Model file for the job. Use its own axes, mm. A direction names the side the tool comes from. Give positions to 0.01 mm unless a question says otherwise; leave off trailing zeros. Write each loop counter-clockwise with the first axis right and the second up, starting at its lowest first coordinate (ties: lowest second). Pieces come first, ordered by that corner, then holes. Notation, with made-up numbers: (67.25, 71.25) - (97.25, 71.25) arc R18 cw to (97.25, 91.25) - close; hole circle Ø1 at (1, 45.25). An arc over 180 degrees is marked (long way). One line per item, written item: value. Start each with the question number.
(1) Cut at A-A, the plane z = 11.25. List the corners of the cut face in (x, y).
(2) Cut at C-C, the plane y = -9.5. List the corners of the cut face in (x, z).
(3) Drop flat-ended pins along their axis: P1, Ø1.9, axis at x = -24.5, y = -4.5, coming from the +Z side; P2, Ø3.5, axis at y = -8.5, z = 6.5, coming from the +X side; P3, Ø2, axis at y = 6, z = 4, coming from the +X side. Give the stop position or say it passes through.
(4) Cut at B-B, the plane x = -8. List the corners of the cut face in (y, z).
(5) Mould opens along X. For faces 5 (the face through (22.4, -14.4, 6.3)), 6 (the face through (22.5, -2, 11)), 7 (the face through (-20.75, 3, 2)) say: pulls with the +X half, pulls with the -X half, needs draft (parallel to the pull), parting line crosses it, or undercut.
(6) Probe L1, parallel to X at y = -22.5, z = 5; L2, parallel to Y at x = -23, z = 5.1; L3, parallel to Y at x = -19, z = 9. List the from-to ranges inside material, lowest first.
(7) 3-axis set-ups, long thin cutter, end or side, ignore diameter. For faces 1 (the face through (-14, -22, 6)), 2 (the face through (-23, 3, 1)), 3 (the face through (-0.4, 20, 26.2)), 4 (the face through (20.28, 4.97, 2.54)): which of +Z, -Z, +X, -X, +Y, -Y reach the whole face in a straight line?
(8) Cut at D-D, the plane x = -23. List the corners of the cut face in (y, z).
from build123d import *

# Parameters (mm, degrees)
SKETCH_1_W             = 56
SKETCH_1_H             = 50
EXTRUDE_487_DEPTH      = 12.5
SKETCH_3_W             = 36
SKETCH_3_H             = 46
CUT_EXTRUDE_730_DEPTH  = 40.563240514
SKETCH_11_R            = 1.25
CUT_EXTRUDE_984_DEPTH  = 10
CUT_EXTRUDE_1451_DEPTH = 8
CUT_EXTRUDE_1793_REACH = 64.588
SKETCH_4_R             = 4.2
SKETCH_6_R             = 4
CUT_EXTRUDE_1930_DEPTH = 10
SKETCH_7_W             = 6.25
SKETCH_7_H             = 20.5
CUT_EXTRUDE_2129_DEPTH = 10
SKETCH_8_R             = 5.25
CUT_EXTRUDE_2306_DEPTH = 2.25
SKETCH_9_R             = 1.1
CUT_EXTRUDE_2664_DEPTH = 5.25
CUT_EXTRUDE_3061_DEPTH = 40.563240514
CHAMFER_1_SIZE         = 1
FILLET_1_R             = 1
SKETCH_12_W            = 20
SKETCH_12_H            = 1.5
CUT_EXTRUDE_3473_DEPTH = 40.563240514
FILLET_2_R             = 0.5
CUT_EXTRUDE_4198_REACH = 41.563
SKETCH_13_W            = 36
SKETCH_13_H            = 1
EXTRUDE_4558_DEPTH     = 5
FILLET_3_R             = 10
FILLET_4_R             = 1.5


with BuildPart() as part:
    # Эскиз1 → Extrude 487 (new body)
    with BuildSketch(Plane.XY):
        Rectangle(SKETCH_1_W, SKETCH_1_H)
    extrude(amount=EXTRUDE_487_DEPTH)

    # Эскиз3 → Cut-Extrude 730 (cut, through all)
    with BuildSketch(Plane.XY.offset(12.5)):
        with Locations((0, 1)):
            Rectangle(SKETCH_3_W, SKETCH_3_H)
    extrude(amount=-CUT_EXTRUDE_730_DEPTH, mode=Mode.SUBTRACT)

    # Эскиз11 → Cut-Extrude 984 (cut)
    with BuildSketch(Plane.XZ.offset(25)):
        with Locations(Location((-25, 5, 0), (0, 0, 270))):
            Circle(SKETCH_11_R)
        with Locations(Location((25, 5, 0), (0, 0, 270))):
            Circle(SKETCH_11_R)
    cut_extrude_984 = extrude(amount=-CUT_EXTRUDE_984_DEPTH, mode=Mode.SUBTRACT)

    # Mirror 1028: Cut-Extrude 984 across plane
    add(cut_extrude_984.mirror(Plane.ZX), mode=Mode.SUBTRACT)

    # Эскиз5 → Cut-Extrude 1451 (cut)
    with BuildSketch(Plane(origin=(28, 0, 0), x_dir=(0, 0, -1), z_dir=(1, 0, 0))):
        with BuildLine():
            Line((-9.688027281, 0.587538929), (-8.743079599, -12.085887362))
            ThreePointArc((-8.743079599, -12.085887362), (-6.25, -14.4), (-3.756920401, -12.085887362))
            Line((-3.756920401, -12.085887362), (-2.811972719, 0.587538929))
            ThreePointArc((-2.811972719, 0.587538929), (-6.25, 7.2), (-9.688027281, 0.587538929))
        make_face()
    extrude(amount=-CUT_EXTRUDE_1451_DEPTH, mode=Mode.SUBTRACT)

    # Эскиз4 → Cut-Extrude 1793 (cut, up to next)
    with BuildSketch(Plane(origin=(28, 0, 0), x_dir=(0, 0, -1), z_dir=(1, 0, 0)), mode=Mode.PRIVATE) as cut_extrude_1793_sk1:
        with Locations((-6.25, 3)):
            Circle(SKETCH_4_R)
    cut_extrude_1793_tool1 = extrude(cut_extrude_1793_sk1.sketch, amount=-CUT_EXTRUDE_1793_REACH, mode=Mode.PRIVATE) & part.part
    add(cut_extrude_1793_tool1.solids().sort_by_distance((28, 3, 6.25))[0], mode=Mode.SUBTRACT)

    # Эскиз6 → Cut-Extrude 1930 (cut)
    with BuildSketch(Plane.ZY.offset(28)):
        with Locations((6.25, 3)):
            Circle(SKETCH_6_R)
    extrude(amount=-CUT_EXTRUDE_1930_DEPTH, mode=Mode.SUBTRACT)

    # Эскиз7 → Cut-Extrude 2129 (cut)
    with BuildSketch(Plane.ZY.offset(28)):
        with Locations((9.375, 3)):
            Rectangle(SKETCH_7_W, SKETCH_7_H)
    extrude(amount=-CUT_EXTRUDE_2129_DEPTH, mode=Mode.SUBTRACT)

    # Эскиз8 → Cut-Extrude 2306 (cut, symmetric)
    with BuildSketch(Plane.ZY.offset(23)):
        with Locations((6.25, 3)):
            Circle(SKETCH_8_R)
    extrude(amount=CUT_EXTRUDE_2306_DEPTH, both=True, mode=Mode.SUBTRACT)

    # Эскиз9 → Cut-Extrude 2664 (cut)
    with BuildSketch(Plane.XY.offset(6.25)):
        with Locations((-23, 10)):
            Circle(SKETCH_9_R)
        with Locations((-23, -4)):
            Circle(SKETCH_9_R)
    extrude(amount=-CUT_EXTRUDE_2664_DEPTH, mode=Mode.SUBTRACT)

    # Эскиз10 → Cut-Extrude 3061 (cut, through all)
    with BuildSketch(Plane.XY.offset(12.5)):
        Polygon((28, -16.3), (28, 12.7), (22.5, 7.2), (22.5, -10.8), align=None)
    extrude(amount=-CUT_EXTRUDE_3061_DEPTH, mode=Mode.SUBTRACT)

    # Фаска1
    chamfer_1_edges = [part.edges().sort_by_distance(p)[0] for p in [
        (-28, 3, 2.25),
        (-18, 3, 2.25),
    ]]
    chamfer(chamfer_1_edges, length=CHAMFER_1_SIZE)

    # Скругление1
    fillet_1_edges = [part.edges().sort_by_distance(p)[0] for p in [
        (18, -22, 6.25),
        (-18, -22, 6.25),
    ]]
    fillet(fillet_1_edges, radius=FILLET_1_R)

    # Эскиз12 → Cut-Extrude 3473 (cut, through all)
    with BuildSketch(Plane.XY):
        with Locations((0, -22.75)):
            Rectangle(SKETCH_12_W, SKETCH_12_H)
    extrude(amount=CUT_EXTRUDE_3473_DEPTH, mode=Mode.SUBTRACT)

    # Скругление2
    fillet_2_edges = [part.edges().sort_by_distance(p)[0] for p in [
        (-10, -22, 6.25),
        (-10, -23.5, 6.25),
        (10, -23.5, 6.25),
        (10, -22, 6.25),
    ]]
    fillet(fillet_2_edges, radius=FILLET_2_R)

    # Эскиз13 → Cut-Extrude 4198 (cut, up to next)
    with BuildSketch(Plane.XY.offset(12.5), mode=Mode.PRIVATE) as cut_extrude_4198_sk1:
        with Locations((0, 24.5)):
            Rectangle(SKETCH_13_W, SKETCH_13_H)
    cut_extrude_4198_tool1 = extrude(cut_extrude_4198_sk1.sketch, amount=-CUT_EXTRUDE_4198_REACH, mode=Mode.PRIVATE) & part.part
    add(cut_extrude_4198_tool1.solids().sort_by_distance((0, 24.5, 12.5))[0], mode=Mode.SUBTRACT)

    # Эскиз14 → Extrude 4558 (add)
    with BuildSketch(Plane(origin=(0, 25, 0), x_dir=(1, 0, 0), z_dir=(0, 1, 0))):
        Polygon((-28, -12.5), (-28, -28), (28, -28), (28, -12.5), (18, -12.5), (18, -24.5), (-18, -24.5), (-18, -12.5), align=None)
    extrude(amount=-EXTRUDE_4558_DEPTH)

    # Скругление3
    # the kernel refuses this fillet: 10 mm, written as the material it adds along each edge
    with BuildSketch(Plane(origin=(28, 20, 12.5), x_dir=(0, -1, 0), z_dir=(-1, 0, 0))) as fillet_3_piece_1_section:
        with BuildLine():
            CenterArc((FILLET_3_R, FILLET_3_R), FILLET_3_R, 180, 90)
            Line((0, FILLET_3_R), (0, 0))
            Line((0, 0), (FILLET_3_R, 0))
        make_face()
    fillet_3_piece_1 = extrude(amount=10, mode=Mode.PRIVATE)
    fillet_3_piece_1 = split(fillet_3_piece_1, bisect_by=Plane(origin=(31.65, 16.35, 12.5), z_dir=(-0.7071067811865515, 0.7071067811865436, 0)), keep=Keep.TOP, mode=Mode.PRIVATE)
    add(fillet_3_piece_1)
    with BuildSketch(Plane(origin=(-18, 20, 12.5), x_dir=(0, -1, 0), z_dir=(-1, 0, 0))) as fillet_3_piece_2:
        with BuildLine():
            CenterArc((10, 9.45714016), FILLET_3_R, 180, 71.034425011)
            Line((0, 9.45714016), (0, 0))
            Line((0, 0), (6.75, 0))
        make_face()
    extrude(amount=10)

    # Скругление4
    fillet_4_edges = [part.edges().sort_by_distance(p)[0] for p in [
        (0, 20, 24.5),
        (0, 20, 28),
        (-28, 22.5, 28),
        (0, 25, 28),
    ]]
    fillet(fillet_4_edges, radius=FILLET_4_R)


solid = part.part
Answers follow:
1. outline: (-28, -25) - (28, -25) - (28, -16.3) - (22.5, -10.8) - (22.5, 7.2) - (28, 12.7) - (28, 25) - (18, 25) - (18, -21) arc R1 cw to (17, -22) - (10.5, -22) arc R0.5 ccw to (10, -22.5) - (10, -23) arc R0.5 cw to (9.5, -23.5) - (-9.5, -23.5) arc R0.5 cw to (-10, -23) - (-10, -22.5) arc R0.5 ccw to (-10.5, -22) - (-17, -22) arc R1 cw to (-18, -21) - (-18, -7.25) - (-28, -7.25) - close; (-28, 13.25) - (-18, 13.25) - (-18, 25) - (-28, 25) - close
2. outline: (-28, 0) - (-18, 0) - (-18, 12.5) - (-28, 12.5) - close; (18, 0) - (22.5, 0) - (22.5, 3.56) - (20, 3.56) - (20, 8.94) - (22.5, 8.94) - (22.5, 12.5) - (18, 12.5) - close
3. P1: stops at z = 6.25
3. P2: stops at x = 20
3. P3: stops at x = 22.5
4. outline: (-25, 0) - (-23.5, 0) - (-23.5, 12.5) - (-25, 12.5) - close; (20, 26) arc R1.5 ccw to (21.5, 24.5) - (25, 24.5) - (25, 26.5) arc R1.5 ccw to (23.5, 28) - (21.5, 28) arc R1.5 ccw to (20, 26.5) - close
5. face 5: needs draft
5. face 6: pulls with the +X half
5. face 7: undercut
6. L1: x = -28 to -26.25, -23.75 to -10, 10 to 23.75, 26.25 to 28
6. L2: y = -25 to -5.1, -2.9 to -2.12, 8.12 to 8.9, 11.1 to 25
6. L3: y = -25 to -7.25, 13.25 to 25
7. face 1: +Z, -Z, +Y
7. face 2: +Z
7. face 3: +Z, +X, -X, -Y
7. face 4: +X
8. outline: (-25, 0) - (25, 0) - (25, 26.5) arc R1.5 ccw to (23.5, 28) - (21.5, 28) arc R1.5 ccw to (20, 26.5) - (20, 21.96) arc R10 cw to (13.25, 12.5) - (13.25, 6.25) - (11.1, 6.25) - (11.1, 1) - (8.9, 1) - (8.9, 6.25) - (8.25, 6.25) arc R5.25 cw to (-2.25, 6.25) - (-2.9, 6.25) - (-2.9, 1) - (-5.1, 1) - (-5.1, 6.25) - (-7.25, 6.25) - (-7.25, 12.5) - (-25, 12.5) - close
